from build123d import *

# Parameters (mm, degrees)
SKETCH1_W               = 35.5
SKETCH1_H               = 28.5
SKETCH1_R               = 1.25
BOSS_EXTRUDE1_DEPTH     = 5
SKETCH2_W               = 25
SKETCH2_H               = 28.5
SKETCH2_R               = 3.5
CUT_EXTRUDE1_DEPTH      = 3
CUT_EXTRUDE2_DEPTH      = 25.74494898
CUT_EXTRUDE2_DEPTH_BACK = 25.74494898
SKETCH3_R               = 3.5
FILLET1_R               = 1
SKETCH4_W               = 30
SKETCH4_H               = 20
BOSS_EXTRUDE5_DEPTH     = 9
CUT_EXTRUDE7_DEPTH      = 34.14079812
CUT_EXTRUDE7_DEPTH_BACK = 34.14079812
CUT_EXTRUDE8_DEPTH      = 36.189664676
CUT_EXTRUDE8_DEPTH_BACK = 36.189664676
SKETCH8_W               = 3
SKETCH8_H               = 3
FILLET2_R               = 2


with BuildPart() as part:
    # Sketch1 → Boss-Extrude1 (new body)
    with BuildSketch(Plane(origin=(0, 0, 0), x_dir=(1, 0, 0), z_dir=(0, 1, 0))):
        with Locations((0, -2.25)):
            Rectangle(SKETCH1_W, SKETCH1_H)
        with Locations(Location((-15, 4.5, 0), (0, 0, 270))):
            Circle(SKETCH1_R, mode=Mode.SUBTRACT)
        with Locations(Location((15, 4.5, 0), (0, 0, 270))):
            Circle(SKETCH1_R, mode=Mode.SUBTRACT)
        with Locations(Location((-15, -12.5, 0), (0, 0, 270))):
            Circle(SKETCH1_R, mode=Mode.SUBTRACT)
        with Locations(Location((15, -12.5, 0), (0, 0, 270))):
            Circle(SKETCH1_R, mode=Mode.SUBTRACT)
    extrude(amount=BOSS_EXTRUDE1_DEPTH)

    # Sketch2 → Cut-Extrude1 (cut)
    with BuildSketch(Plane(origin=(0, 5, 0), x_dir=(1, 0, 0), z_dir=(0, 1, 0))):
        with Locations((0, -2.25)):
            Rectangle(SKETCH2_W, SKETCH2_H)
        with Locations(Location((0, 0, 0), (0, 0, 270))):
            Circle(SKETCH2_R, mode=Mode.SUBTRACT)
    extrude(amount=-CUT_EXTRUDE1_DEPTH, mode=Mode.SUBTRACT)

    # Sketch3 → Cut-Extrude2 (cut, two sides: drawn at the far end of the back side and taken through both)
    with BuildSketch(Plane(origin=(0, 5, 0), x_dir=(1, 0, 0), z_dir=(0, 1, 0)).offset(-CUT_EXTRUDE2_DEPTH_BACK)):
        with Locations(Location((0, 0, 0), (0, 0, 270))):
            Circle(SKETCH3_R)
    extrude(amount=CUT_EXTRUDE2_DEPTH + CUT_EXTRUDE2_DEPTH_BACK, mode=Mode.SUBTRACT)

    # Fillet1
    fillet1_edges = [part.edges().sort_by_distance(p)[0] for p in [
        (12.5, 2, 2.25),
        (-12.5, 2, 2.25),
    ]]
    fillet(fillet1_edges, radius=FILLET1_R)

    # Sketch4 → Boss-Extrude5 (add)
    with BuildSketch(Plane.XZ):
        Rectangle(SKETCH4_W, SKETCH4_H)
    extrude(amount=BOSS_EXTRUDE5_DEPTH)

    # Sketch7 → Cut-Extrude7 (cut, two sides: drawn at the far end of the back side and taken through both)
    with BuildSketch(Plane(origin=(0, 0, -10), x_dir=(-1, 0, 0), z_dir=(0, 0, -1)).offset(-CUT_EXTRUDE7_DEPTH_BACK)):
        Polygon((12, -6), (12, -9), (15, -9), (15, 0), (9, 0), (9, -6), align=None)
        Polygon((-15, -9), (-12, -9), (-12, -6), (-9, -6), (-9, 0), (-15, 0), align=None)
    extrude(amount=CUT_EXTRUDE7_DEPTH + CUT_EXTRUDE7_DEPTH_BACK, mode=Mode.SUBTRACT)

    # Sketch8 → Cut-Extrude8 (cut, two sides: drawn at the far end of the back side and taken through both)
    with BuildSketch(Plane.ZY.offset(12).offset(-CUT_EXTRUDE8_DEPTH_BACK)):
        with Locations((0, -7.5)):
            Rectangle(SKETCH8_W, SKETCH8_H)
    extrude(amount=CUT_EXTRUDE8_DEPTH + CUT_EXTRUDE8_DEPTH_BACK, mode=Mode.SUBTRACT)

    # Fillet2
    # the kernel refuses this fillet: 2 mm, written as the material it adds along each edge
    with BuildSketch(Plane(origin=(9, 0, -10), x_dir=(1, 0, 0), z_dir=(0, 0, 1))) as fillet2_piece_1:
        with BuildLine():
            CenterArc((FILLET2_R, -FILLET2_R), FILLET2_R, 90, 90)
            Line((0, -FILLET2_R), (0, 0))
            Line((0, 0), (FILLET2_R, 0))
        make_face()
    extrude(amount=20)
    with BuildSketch(Plane(origin=(-9, 0, -10), x_dir=(-1, 0, 0), z_dir=(0, 0, 1))) as fillet2_piece_2:
        with BuildLine():
            CenterArc((FILLET2_R, FILLET2_R), FILLET2_R, 180, 90)
            Line((0, FILLET2_R), (0, 0))
            Line((0, 0), (FILLET2_R, 0))
        make_face()
    extrude(amount=20)
    with BuildSketch(Plane(origin=(-9, -6, -1.5), x_dir=(0, 0, 1), z_dir=(1, 0, 0)), Plane(origin=(9, -6, 1.5), x_dir=(0, 0, -1), z_dir=(-1, 0, 0))) as fillet2_piece_3:
        with BuildLine():
            CenterArc((FILLET2_R, FILLET2_R), FILLET2_R, 180, 90)
            Line((0, FILLET2_R), (0, 0))
            Line((0, 0), (FILLET2_R, 0))
        make_face()
    extrude(amount=18)


solid = part.part
Build history of the part. All positions in model axes, mm. A direction names the side the tool comes from. Coordinates: 2 decimals unless noted, no trailing zeros. Write each loop counter-clockwise with the first axis right and the second up, starting at its lowest first coordinate (ties: lowest second). Pieces come first, ordered by that corner, then holes. Notation, with made-up numbers: (75, 65.25) -> (94, 65.25) arc R16 ccw to (94, 83.25) -> close; hole circle Ø2 at (-32.75, 36.5). An arc over 180 degrees is marked (long way). Use CSV: the item, a comma, the result in double quotes. Start each with the question number.
Q1. Pull direction Z, two halves, no side cores. Call faces 1 (the flat face through (0, 1, 16.5)), 2 (the flat face through (0.2, -8.2, 1.5)), 3 (the flat face through (0, -5, -10)), 4 (the flat face through (-10, -6, 6)): released by +Z, released by -Z, zero draft, split by the parting line, or undercut.
Q2. Drill centre lines: probe 1 along X at (y, z) = (1.95, -4.5); probe 2 along X at (y, z) = (2.9, -4.5); probe 3 along Z at (x, y) = (-2.5, -8). Where is each one in solid material? Low to high.
Q3. Cut at A-A, the plane z = 12.5. List the corners of the cut face in (x, y).
Q4. Cut at C-C, the plane x = -6. List the corners of the cut face in (y, z), then the cut area to 3 significant figures.
Q5. Cut at D-D, the plane z = -7.75. List the corners of the cut face in (x, y), then the cut area to 3 significant figures.
Q6. Cut at B-B, the plane x = 15. List the corners of the cut face in (y, z).
Q7. 3-axis set-ups, long thin cutter, end or side, ignore diameter. For faces 5 (the flat face through (11, -6, -6)), 6 (the flat face through (-12.5, 4, 2)), 7 (the flat face through (0.2, -8.2, -1.5)), 8 (the cylindrical face through (-0.1, -6.8, -1.1)), 9 (the flat face through (12, -8, 6)): which of +Z, -Z, +X, -X, +Y, -Y reach the whole face in a straight line?
Q8. Flat gauge pins, fed straight in: pin 1 Ø5 at (y, z) = (-3.5, 10.5) entering from +X; pin 2 Ø3 at (x, z) = (-15, -4.5) entering from -Y; pin 3 Ø7 at (x, y) = (1.5, -4.5) entering from +Z. Where does each tip first touch, or does it go through?
Checked values:
1,face 1,"released by +Z"
1,face 2,"undercut"
1,face 3,"released by -Z"
1,face 4,"zero draft"
2,probe 1,"x = -17.75 to -16.25, -13.75 to 13.75, 16.25 to 17.75"
2,probe 2,"x = -17.75 to -16.25, -13.75 to -12.49, 12.49 to 13.75, 16.25 to 17.75"
2,probe 3,"z = -10 to -1.5, 1.5 to 10"
3,outline,"(-17.75, 0) -> (-16.25, 0) -> (-16.25, 5) -> (-17.75, 5) -> close; (-13.75, 0) -> (13.75, 0) -> (13.75, 5) -> (12.5, 5) -> (12.5, 3) arc R1 cw to (11.5, 2) -> (-11.5, 2) arc R1 cw to (-12.5, 3) -> (-12.5, 5) -> (-13.75, 5) -> close; (16.25, 0) -> (17.75, 0) -> (17.75, 5) -> (16.25, 5) -> close"
4,outline,"(-9, -10) -> (0, -10) -> (0, -12) -> (2, -12) -> (2, 16.5) -> (0, 16.5) -> (0, 10) -> (-9, 10) -> (-9, 1.5) -> (-8, 1.5) arc R2 cw to (-6.06, 0) arc R2 cw to (-8, -1.5) -> (-9, -1.5) -> close"
4,area,"230 mm²"
5,outline,"(-17.75, 0) -> (-11, 0) arc R2 cw to (-9, -2) -> (-9, -6) -> (-12, -6) -> (-12, -9) -> (12, -9) -> (12, -6) -> (9, -6) -> (9, -2) arc R2 cw to (11, 0) -> (17.75, 0) -> (17.75, 5) -> (12.5, 5) -> (12.5, 3) arc R1 cw to (11.5, 2) -> (-11.5, 2) arc R1 cw to (-12.5, 3) -> (-12.5, 5) -> (-17.75, 5) -> close"
5,area,"285 mm²"
6,outline,"(0, -12) -> (5, -12) -> (5, -5.75) -> (0, -5.75) -> close; (0, -3.25) -> (5, -3.25) -> (5, 11.25) -> (0, 11.25) -> close; (0, 13.75) -> (5, 13.75) -> (5, 16.5) -> (0, 16.5) -> close"
7,face 5,"+Z, -Z, +X"
7,face 6,"+Z, -Z, +Y"
7,face 7,"-Y"
7,face 8,"+X, -X, -Y"
7,face 9,"+Z, -Z, +X, -Y"
8,pin 1,"stops at x = 9.24"
8,pin 2,"stops at y = 0"
8,pin 3,"stops at z = 10"
